Model file for the job. Use its own axes, mm. Face numbers are marked on the shaded views. A direction names the side the tool comes from. Round coordinates to 2 decimals unless told otherwise and drop trailing zeros. Order: outer loops, then holes, each group sorted by start corner. A loop starts at its lowest first (then second) coordinate and runs counter-clockwise, first axis right, second up. Notation, with made-up numbers: (58, 6.25) -> (79, 6.25) arc R18 ccw to (79, 18.25) -> close; hole circle Ø1 at (-7.75, -22.75). An arc over 180 degrees is marked (long way). Answer as CSV lines item,"result".
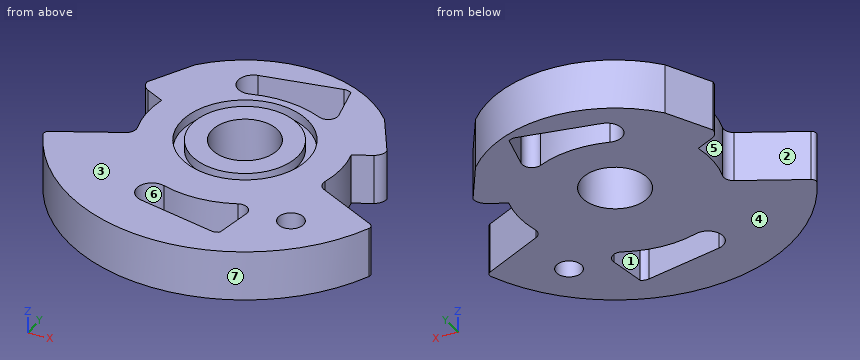
Autodesk Inventor part; units mm, degrees
ref_plane "Arbeitsebene1" through (0, 0, 0) normal (1, 0, 0) x (0, 1, 0)
ref_plane "Arbeitsebene2" through (0, -3, 0) normal (0, 1, 0) x (-1, 0, 0)
ref_plane "XY Plane" through (0, 0, 0) normal (0, 0, 1) x (1, 0, 0)
sketch "Skizze1" plane through (0, 0, 0) normal (0, 0, 1) x (1, 0, 0)
  line L0 (0, 25) -> (0, -35) construction
  line L1 (-32.2, 0) -> (32.2, 0) construction
  circle A0 centre (0, 0) radius 19
  line L2 (-18.5027, 4.3188) -> (-24, 7)
  line L3 (-17.7846, -6.6863) -> (-32.2, -13.7171)
  line L4 (18.5027, 4.3188) -> (24, 7)
  line L5 (17.7846, -6.6863) -> (32.2, -13.7171)
  arc A1 (-32.2, -13.7171) -> (32.2, -13.7171) centre (0, 0) ccw
  arc A2 (24, 7) -> (-24, 7) centre (0, 0) ccw
  dimension "d3" = 38
  dimension "d4" = 26
  dimension "d5" = 52
  dimension "d6" = 26
  dimension "d7" = 52
  dimension "d8" = 48
  dimension "d9" = 64.4
  dimension "d10" = 60
  dimension "d11" = 25
extrude "Extrusion1" add sketch "Skizze1" along normal blind 10
fillet "Rundung1" radius 2.5 2 edges at (24, 7, 5) (-24, 7, 5)
sketch "Skizze2" plane through (0, 0, 10) normal (0, 0, 1) x (1, 0, 0)
  line L0 (0, 0) -> (24.7487, -24.7487) construction
  arc A0 (-32.2, -13.7171) -> (32.2, -13.7171) centre (0, 0) ccw
  line L1 (0, 0) -> (35, 0) construction
  point P0 (18.7383, -18.7383)
  dimension "d15" = 45
  dimension "d16" = 26.5
hole "Bohrung1" at (18.7383, -18.7383, 10) direction (0, 0, -1) diameter 5 end through all
fillet "Rundung2" radius 1 2 edges at (32.2, -13.7171, 5) (-32.2, -13.7171, 5)
fillet "Rundung3" radius 2 2 edges at (17.7846, -6.6863, 5) (-17.7846, -6.6863, 5)
sketch "Skizze3" plane through (0, 0, 10) normal (0, 0, 1) x (1, 0, 0)
  arc A0 (-23.2457, 9.1998) -> (-22.0171, 6.0329) centre (-20.9211, 8.2798) ccw
  line L0 (-23.4211, 8.2798) -> (-23.4211, 29.6928) construction
  line L1 (-23.4211, 8.2798) -> (-18.4816, 16.8354)
  line L2 (-23.4211, 8.2798) -> (-11.3111, 8.2798) construction
  arc A1 (23.2457, 9.1998) -> (-23.2457, 9.1998) centre (0, 0) ccw
  dimension "d27" = 30
extrude "Extrusion2" cut sketch "Skizze3" against normal through all
ref_plane "Arbeitsebene1" through (0, 0, 0) normal (1, 0, 0) x (0, 1, 0)
mirror "Spiegeln1" about plane through (0, 0, 0) normal (1, 0, 0) of "Extrusion2"
sketch "Skizze4" plane through (0, 0, 10) normal (0, 0, 1) x (1, 0, 0)
  circle A0 centre (0, 0) radius 6.5
  dimension "d31" = 13
extrude "Extrusion3" cut sketch "Skizze4" against normal blind 10
sketch "Skizze5" plane through (0, 0, 10) normal (0, 0, 1) x (1, 0, 0)
  circle A0 centre (0, 0) radius 10.5
  circle A1 centre (0, 0) radius 12.5
  dimension "d34" = 21
  dimension "d35" = 25
extrude "Extrusion4" cut sketch "Skizze5" against normal blind 2
sketch "Skizze6" plane through (0, 0, 10) normal (0, 0, 1) x (1, 0, 0)
  arc A0 (-5.8207, -19.1299) -> (-7.2677, -24.9446) centre (-6.694, -22) ccw
  line L0 (-7.2677, -24.9446) -> (7.9346, -27.9063)
  arc A1 (7.9346, -27.9063) -> (9.4512, -27.5686) centre (8.306, -26) ccw
  line L1 (9.4512, -27.5686) -> (10.8468, -20.405)
  arc A2 (10.8468, -20.405) -> (8.1489, -18.2601) centre (8.9404, -20.0336) ccw
  arc A3 (-5.8207, -19.1299) -> (8.1489, -18.2601) centre (0, 0) ccw
  circle A4 centre (0, 0) radius 12.5
  line L2 (0, 0) -> (0, -16.1046) construction
  dimension "d38" = 15
  dimension "d40" = 6
  dimension "d41" = 3
  dimension "d42" = 19.9959
  dimension "d43" = 22
  dimension "d44" = 26
  dimension "d45" = 20.0336
extrude "Extrusion5" cut sketch "Skizze6" against normal up to surface (10 mm away) contours A3 A2 L1 A1 L0 A0
ref_plane "Arbeitsebene2" through (0, -3, 0) normal (0, 1, 0) x (-1, 0, 0)
mirror "Spiegeln2" about plane through (0, -3, 0) normal (0, 1, 0) of "Extrusion5"
properties part number "disc" material "Stahl, galvanisiert"
Q1. Flat gauge pins, fed straight in: pin 1 (1 mm diameter, centred on x = 9.5, z = 2, fed in from +Y); pin 2 (5 mm diameter, centred on y = 6.5, z = 6, fed in from +X); pin 3 (22.5 mm diameter, centred on x = 0, y = 0, fed in from -Z); pin 4 (1.5 mm diameter, centred on y = -25.5, z = 6.5, fed in from +X). Where does each tip first touch, or does it go through?
Checks:
pin 1,"y = 23.32"
pin 2,"x = 23.42"
pin 3,"z = 0"
pin 4,"x = 24.75"
Q2. Saw through at A-A (y = 0). Write the cut outline in (x, z).
Checks:
outline,"(-19, 0) -> (-6.5, 0) -> (-6.5, 10) -> (-10.5, 10) -> (-10.5, 8) -> (-12.5, 8) -> (-12.5, 10) -> (-19, 10) -> close; (6.5, 0) -> (19, 0) -> (19, 10) -> (12.5, 10) -> (12.5, 8) -> (10.5, 8) -> (10.5, 10) -> (6.5, 10) -> close"
Q3. Tool access for the marked faces 1, 2 and 3: list every direction of +Z, -Z, +X, -X, +Y, -Y with a clear straight run to the whole face (end or side of a thin tool).
Checks:
face 1,"+Z, -Z"
face 2,"+Z, -Z, -X"
face 3,"+Z, +X, -X, +Y, -Y"
Q4. Saw through at B-B (z = 9). State how many separate pieces and enclosed holes the cut face has, plus the area to 3 significant figures.
Checks:
separate pieces,"2"
enclosed holes,"5"
area,"1,920 mm²"
Q5. Wall check: L1, parallel to Y at x = 0, z = 8.95; L2, parallel to Y at x = 1, z = 4; L3, parallel to X at y = 15.5, z = 7.5. Give the ranges that are in metal, low to high. Write a range as [from, to].
Checks:
L1,"[-35, -26.36], [-20, -12.5], [-10.5, -6.5], [6.5, 10.5], [12.5, 14], [20.36, 25]"
L2,"[-34.99, -26.56], [-19.97, -6.42], [6.42, 13.97], [20.56, 24.98]"
L3,"[-19.25, -9.65], [10.63, 19.25]"
Q6. Saw through at C-C (x = 0.5). Write the cut outline in (y, z) (3 decimals), plus the area to 3 significant figures.
Checks:
outline,"(-34.996, 0) -> (-26.458, 0) -> (-26.458, 10) -> (-34.996, 10) -> close; (-19.99, 0) -> (-6.481, 0) -> (-6.481, 10) -> (-10.488, 10) -> (-10.488, 8) -> (-12.49, 8) -> (-12.49, 10) -> (-19.99, 10) -> close; (6.481, 0) -> (13.99, 0) -> (13.99, 10) -> (12.49, 10) -> (12.49, 8) -> (10.488, 8) -> (10.488, 10) -> (6.481, 10) -> close; (20.458, 0) -> (24.995, 0) -> (24.995, 10) -> (20.458, 10) -> close"
area,"333 mm²"
Q7. Mould opens along Y. For the marked faces 4, 5, 6 and 7 say: +Y half, -Y half, draft (parallel to the pull), parting line (faces both ways), or undercut.
Checks:
face 4,"draft"
face 5,"undercut"
face 6,"undercut"
face 7,"-Y half"
